Design review of the part built by this model. Coordinates are the model's own, in mm. A direction names the side the tool comes from. Coordinates: 2 decimals unless noted, no trailing zeros. Write each loop counter-clockwise with the first axis right and the second up, starting at its lowest first coordinate (ties: lowest second). Pieces come first, ordered by that corner, then holes. Notation, with made-up numbers: (21.5, 16.5) - (78.5, 16.5) arc R27 cw to (78.5, 33.5) - close; hole circle Ø6 at (66.5, 12). An arc over 180 degrees is marked (long way). Answer as CSV lines item,"result". Start each with the question number.
Q1. Mouldability with a two-part tool opening along Y and no side actions: class faces 1 (the face through (77.27, 0.91, -75.25)), 2 (the face through (100, 1.6, -13.4)), 3 (the face through (77.27, 4.13, -4.08)) as pulls with the +Y half, pulls with the -Y half, needs draft (parallel to the pull), parting line crosses it, or undercut.
Q2. We need section D-D (y = 24.5). Write out the cut boundary in (x, z) (3 decimals), plus the area to 3 significant figures.
Q3. Clearance check with flat-ended pins moving along their axes: pin 1 (5.5 mm diameter, centred on x = 12.5, z = -15, fed in from +Y) (3 decimals); pin 2 (4 mm diameter, centred on x = 8, y = 15.4, fed in from +Z). State where each tip first meets the part, or that it passes through.
Q4. We need section C-C (z = -44.5). Write out the cut boundary in (x, y) (3 decimals).
Q5. We need section B-B (x = 50). Write out the cut boundary in (y, z) (3 decimals).
Q6. For line 1 along X through (y, z) = (50.2, -57.35) (3 decimals); line 2 along Y through (x, z) = (65, -25.5) (3 decimals); line 3 along X through (y, z) = (48, -15) (3 decimals), list the stretches that pass through material, from the lowest coordinate up. Write a range as [from, to].
Q7. We need section A-A (y = 15.4). Write out the cut boundary in (x, z) (3 decimals).
Q8. Machinability: for faces 4 (the face through (52.21, 1.57, -66.63)), 5 (the face through (101.453, 49.235, -19.804)), 6 (the face through (75, 25, -3.175)), which of the approach directions +Z, -Z, +X, -X, +Y, -Y give a long, thin tool a straight path to every point of the face, cutting with its end or side? Answer none if there is none.
Autodesk Inventor part; units mm, degrees
ref_plane "Work Plane1" through (76.2, 0, 0) normal (1, 0, 0) x (0, 0, -1)
ref_plane "YZ Plane" through (0, 0, 0) normal (1, 0, 0) x (0, 1, 0)
ref_plane "XZ Plane" through (0, 0, 0) normal (0, 1, 0) x (-1, 0, 0)
sketch "Sketch1" plane through (0, 0, 0) normal (1, 0, 0) x (0, 1, 0)
  line L0 (0, 0) -> (50.8, 0)
  line L1 (50.8, 0) -> (50.8, -76.2)
  line L2 (50.8, -76.2) -> (0, -76.2)
  line L3 (0, -76.2) -> (0, 0)
  dimension "d0" = 76.2
  dimension "d1" = 50.8
extrude "Extrusion1" add sketch "Sketch1" along normal blind 152.4
shell "Shell1" thickness 3.175 removed faces 2 at (0, 33.8667, -50.8) at (152.4, 33.8667, -50.8)
fillet "Fillet1" radius 3.175 8 edges at (76.2, 50.8, -76.2) (76.2, 50.8, 0) (76.2, 0, -76.2) (76.2, 0, 0) (76.2, 3.175, -3.175) (76.2, 3.175, -73.025) (76.2, 47.625, -3.175) (76.2, 47.625, -73.025)
sketch "Sketch2" plane through (0, 0, -73.025) normal (0, -1, 0) x (1, 0, 0)
  circle A0 centre (142.4, 61.425) radius 3
  line L0 (142.4, 61.425) -> (102.4, 61.425) construction
  line L1 (102.4, 61.425) -> (102.4, 8.425) construction
  line L2 (102.4, 8.425) -> (142.4, 8.425) construction
  line L3 (142.4, 8.425) -> (142.4, 61.425) construction
  line L4 (152.4, 69.85) -> (152.4, 0) construction
  line L5 (152.4, 66.675) -> (152.4, 3.175) construction
  line L6 (152.4, 34.925) -> (142.4, 34.925) construction
  circle A1 centre (142.4, 8.425) radius 3
  circle A2 centre (102.4, 61.425) radius 3
  circle A3 centre (102.4, 8.425) radius 3
  point P0 (0, 73.025)
  dimension "d6" = 6
  dimension "d7" = 53
  dimension "d8" = 40
  dimension "d9" = 10
ref_plane "Work Plane1" through (76.2, 0, 0) normal (1, 0, 0) x (0, 0, -1)
extrude "Extrusion2" cut sketch "Sketch2" against normal up to surface (3.175 mm away)
mirror "Mirror1" about plane through (76.2, 0, 0) normal (1, 0, 0) of "Extrusion2"
sketch "Sketch3" plane through (0, 50.8, -3.175) normal (0, 1, 0) x (1, 0, 0)
  line L0 (12.5, 58.025) -> (38.3, 58.025) construction
  line L1 (38.3, 58.025) -> (38.3, 11.825) construction
  line L2 (38.3, 11.825) -> (12.5, 11.825) construction
  line L3 (12.5, 11.825) -> (12.5, 58.025) construction
  circle A0 centre (12.5, 58.025) radius 3.175
  circle A1 centre (38.3, 58.025) radius 3.175
  circle A2 centre (12.5, 11.825) radius 3.175
  circle A3 centre (38.3, 11.825) radius 3.175
  line L4 (0, -3.175) -> (50.8, -3.175) construction
  line L5 (50.8, -3.175) -> (50.8, 73.025) construction
  line L6 (50.8, 73.025) -> (0, 73.025) construction
  line L7 (0, 73.025) -> (0, -3.175) construction
  line L8 (38.3, 34.925) -> (50.8, 34.925) construction
  line L9 (25.4, 58.025) -> (25.4, 73.025) construction
  dimension "d12" = 6.35
  dimension "d13" = 50.8
  dimension "d14" = 76.2
  dimension "d16" = 15
  dimension "d17" = 12.5
extrude "Extrusion3" cut sketch "Sketch3" against normal up to surface (3.175 mm away)
sketch "Sketch4" plane through (0, 50.8, -3.175) normal (0, 1, 0) x (1, 0, 0)
  line L0 (50.8, -3.175) -> (152.4, -3.175) construction
  line L1 (152.4, -3.175) -> (152.4, 73.025) construction
  line L2 (152.4, 73.025) -> (50.8, 73.025) construction
  line L3 (50.8, 73.025) -> (50.8, -3.175) construction
  line L4 (152.4, 66.675) -> (50.8, 66.675) construction
  line L5 (50.8, 66.675) -> (50.8, 3.175) construction
  line L6 (50.8, 3.175) -> (152.4, 3.175) construction
  line L7 (152.4, 3.175) -> (152.4, 66.675) construction
  line L8 (101.6, 66.675) -> (101.6, 73.025) construction
  line L9 (101.6, 3.175) -> (101.6, -3.175) construction
  line L10 (72.15, 54.175) -> (124.7, 54.175) construction
  line L11 (124.7, 54.175) -> (124.7, 15.675) construction
  line L12 (124.7, 15.675) -> (72.15, 15.675) construction
  line L13 (72.15, 15.675) -> (72.15, 54.175) construction
  circle A0 centre (72.15, 54.175) radius 3.175
  circle A1 centre (72.15, 15.675) radius 3.175
  circle A2 centre (98.425, 15.675) radius 3.175
  circle A3 centre (98.425, 54.175) radius 3.175
  circle A4 centre (124.7, 54.175) radius 3.175
  circle A5 centre (124.7, 15.675) radius 3.175
  line L14 (57.15, 66.675) -> (57.15, 3.175) construction
  line L15 (57.15, 34.925) -> (72.15, 34.925) construction
  line L16 (124.7, 34.925) -> (139.7, 34.925) construction
  line L17 (139.7, 3.175) -> (139.7, 66.675) construction
  point P0 (0, -3.175)
  dimension "d20" = 101.6
  dimension "d21" = 76.2
  dimension "d22" = 50.8
  dimension "d23" = 63.5
  dimension "d24" = 6.35
  dimension "d25" = 6.35
  dimension "d26" = 12.5
  dimension "d27" = 15
  dimension "d31" = 88.9
extrude "Extrusion4" cut sketch "Sketch4" against normal up to surface (3.175 mm away)
sketch "Sketch5" plane through (0, 3.175, -76.2) normal (0, 0, -1) x (-1, 0, 0)
  circle A0 centre (-8, 32.225) radius 3.175
  circle A1 centre (-8, 12.225) radius 3.175
  line L0 (0, -3.175) -> (-16, -3.175) construction
  line L1 (-16, -3.175) -> (-16, 47.625) construction
  line L2 (-16, 47.625) -> (0, 47.625) construction
  line L3 (0, 47.625) -> (0, -3.175) construction
  line L4 (-8, 32.225) -> (-8, 47.625) construction
  line L5 (-8, 12.225) -> (-8, -3.175) construction
  dimension "d32" = 50.8
  dimension "d33" = 16
  dimension "d34" = 6.35
  dimension "d35" = 20
extrude "Extrusion5" cut sketch "Sketch5" against normal through all
mirror "Mirror2" about plane through (76.2, 0, 0) normal (1, 0, 0) of "Extrusion5"
equation "\"BendRadius\" = Thickness"
equation "\"BendReliefWidth\" = Thickness"
equation "\"BendReliefDepth\" = 0.5 * Thickness"
equation "\"CornerReliefSize\" = 4 * Thickness"
equation "\"MinimumRemnant\" = 2 * Thickness"
equation "\"TransitionRadius\" = BendRadius"
equation "\"JacobiRadiusSize\" = BendRadius"
equation "\"GapSize\" = Thickness"
properties part number "3x6_Bar" material "Steel, Mild"
Results list:
1,face 1,"pulls with the -Y half"
1,face 2,"needs draft"
1,face 3,"undercut"
2,outline,"(0, -76.2) - (152.4, -76.2) - (152.4, -73.025) - (0, -73.025) - close; (0, -3.175) - (152.4, -3.175) - (152.4, 0) - (0, 0) - close"
2,area,"968 mm2"
3,pin 1,"stops at y = 3.175"
3,pin 2,"passes through"
4,outline,"(0, 0) - (152.4, 0) - (152.4, 3.175) - (0, 3.175) - close; (0, 47.625) - (152.4, 47.625) - (152.4, 50.8) - (0, 50.8) - close"
5,outline,"(0, -73.025) arc R3.175 ccw to (3.175, -76.2) - (47.625, -76.2) arc R3.175 ccw to (50.8, -73.025) - (50.8, -3.175) arc R3.175 ccw to (47.625, 0) - (3.175, 0) arc R3.175 ccw to (0, -3.175) - (0, -8.6) - (3.175, -8.6) - (3.175, -6.35) arc R3.175 cw to (6.35, -3.175) - (44.45, -3.175) arc R3.175 cw to (47.625, -6.35) - (47.625, -69.85) arc R3.175 cw to (44.45, -73.025) - (6.35, -73.025) arc R3.175 cw to (3.175, -69.85) - (3.175, -67.6) - (0, -67.6) - close; (0, -61.6) - (3.175, -61.6) - (3.175, -14.6) - (0, -14.6) - close"
6,line 1,"x = [0, 68.975], [75.325, 95.25], [101.6, 121.525], [127.875, 152.4]"
6,line 2,"y = [0, 3.175], [47.625, 50.8]"
6,line 3,"x = [0, 9.325], [15.675, 35.125], [41.475, 152.4]"
7,outline,"(0, -76.2) - (4.825, -76.2) - (4.825, -73.025) - (0, -73.025) - close; (0, -3.175) - (4.825, -3.175) - (4.825, 0) - (0, 0) - close; (11.175, -76.2) - (141.225, -76.2) - (141.225, -73.025) - (11.175, -73.025) - close; (11.175, -3.175) - (141.225, -3.175) - (141.225, 0) - (11.175, 0) - close; (147.575, -76.2) - (152.4, -76.2) - (152.4, -73.025) - (147.575, -73.025) - close; (147.575, -3.175) - (152.4, -3.175) - (152.4, 0) - (147.575, 0) - close"
8,face 4,"-Y"
8,face 5,"+Y"
8,face 6,"+X, -X"
